Here's how the part is built. I have some questions about the finished solid (model axes, mm). Face numbers are marked on the shaded views. A direction names the side the tool comes from. Round coordinates to 2 decimals unless told otherwise and drop trailing zeros. Order: outer loops, then holes, each group sorted by start corner. A loop starts at its lowest first (then second) coordinate and runs counter-clockwise, first axis right, second up. Notation, with made-up numbers: (42.5, 76) -> (97.5, 76) arc R28 cw to (97.5, 108) -> close; hole circle Ø5 at (52.25, -14). An arc over 180 degrees is marked (long way). One line per item, written item: value.
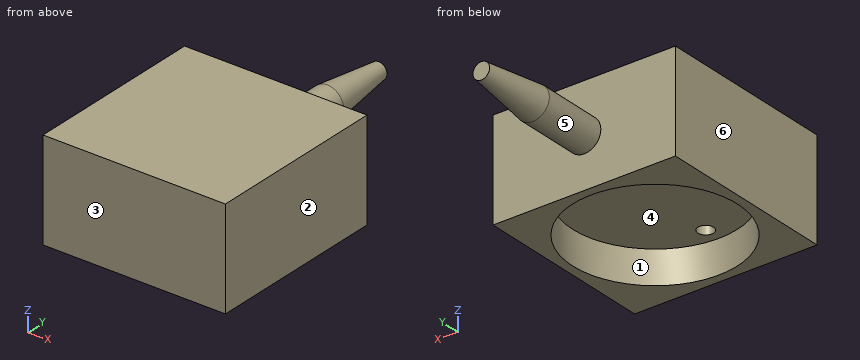
```python
from build123d import *

# Parameters (mm, degrees)
F2_W     = 69.85
F2_H     = 38.1
F3_DEPTH = 69.85
F4_R     = 3
F4_R_2   = 31.5
F5_DEPTH = 12.7
F6_DEPTH = 25.4


with BuildPart() as f1:
    # F0 (on Right) → F1 (revolve)
    with BuildSketch(Plane.YZ):
        Polygon((0, 6.35), (0, 0), (50.8, 0), (50.8, 3.175), (25.4, 6.35), align=None)
    revolve(axis=Axis((0, 25.4, 0), (0, 1, 0)))

    # F2 (on Front) → F3 (join)
    with BuildSketch(Plane.XZ):
        Rectangle(F2_W, F2_H)
    extrude(amount=F3_DEPTH)

    # F4 (on face) → F5 (cut)
    with BuildSketch(Plane(origin=(0, 0, -19.05), x_dir=(1, 0, 0), z_dir=(0, 0, -1))):
        with Locations((0, 59.925)):
            Circle(F4_R)
        with Locations((0, 34.925)):
            Circle(F4_R_2)
        with Locations((0, 59.925)):
            Circle(F4_R, mode=Mode.SUBTRACT)
    extrude(amount=-F5_DEPTH, mode=Mode.SUBTRACT)

    # F4 (on face) → F6 (cut)
    with BuildSketch(Plane(origin=(0, 0, -19.05), x_dir=(1, 0, 0), z_dir=(0, 0, -1))):
        with Locations((0, 59.925)):
            Circle(F4_R)
    extrude(amount=-F6_DEPTH, mode=Mode.SUBTRACT)


solid = f1.part
```
Q1. For P1, Ø4, axis at y = 13, z = 2.5, coming from the -X side; P2, Ø5, axis at y = 10.5, z = -1, coming from the +X side; P3, Ø5, axis at x = 17, z = 15, coming from the +Y side, each with a flat end and sliding along its axis, tell me the tip position at first contact or that it passes through.
Answers:
P1: x = -6.33
P2: x = 6.35
P3: y = 0
Q2. I want a section at C-C on y = -45. Write out the boundary of the cut face in (x, z) (3 decimals), then the cut area to 3 significant figures.
Answers:
outline: (-34.925, -19.05) -> (-29.845, -19.05) -> (-29.845, -6.35) -> (29.845, -6.35) -> (29.845, -19.05) -> (34.925, -19.05) -> (34.925, 19.05) -> (-34.925, 19.05) -> close
area: 1,900 mm2
Q3. I need wall thicknesses on line 1 along Y through (x, z) = (0, 0) (3 decimals); line 2 along X through (y, z) = (-35.5, -17) (3 decimals); line 3 along Y through (x, z) = (-6, 17). Which ranges of each line are inside material? Lowest first, please.
Answers:
line 1: -69.85 to -62.925, -56.925 to 50.8
line 2: -34.925 to -31.495, 31.495 to 34.925
line 3: -69.85 to 0
Q4. I want a section at A-A on x = 0. Write out the boundary of the cut face in (y, z) (3 decimals).
Answers:
outline: (-69.85, -19.05) -> (-66.425, -19.05) -> (-66.425, -6.35) -> (-62.925, -6.35) -> (-62.925, 6.35) -> (-56.925, 6.35) -> (-56.925, -6.35) -> (-3.425, -6.35) -> (-3.425, -19.05) -> (0, -19.05) -> (0, -6.35) -> (25.4, -6.35) -> (50.8, -3.175) -> (50.8, 3.175) -> (25.4, 6.35) -> (0, 6.35) -> (0, 19.05) -> (-69.85, 19.05) -> close
Q5. I want a section at D-D on x = -20. Write out the boundary of the cut face in (y, z).
Answers:
outline: (-69.85, -19.05) -> (-59.26, -19.05) -> (-59.26, -6.35) -> (-10.59, -6.35) -> (-10.59, -19.05) -> (0, -19.05) -> (0, 19.05) -> (-69.85, 19.05) -> close
Q6. If we mould it in two halves opening along X, with no side actions, what happens to the marked faces 1, 2 and 3? For each: pulls with the +X half, pulls with the -X half, needs draft (parallel to the pull), parting line crosses it, or undercut.
Answers:
face 1: undercut
face 2: pulls with the +X half
face 3: needs draft
Q7. Which directions (+Z, -Z, +X, -X, +Y, -Y) give clear straight access to the entire face, cutting with the end or side of a thin tool? Please do the marked faces 4, 5 and 6.
Answers:
face 4: -Z
face 5: +Y
face 6: +Z, -Z, -X, +Y, -Y
Q8. I want a section at B-B on z = -11.5. Write out the boundary of the cut face in (x, y) (3 decimals).
Answers:
outline: (-34.925, -69.85) -> (34.925, -69.85) -> (34.925, 0) -> (-34.925, 0) -> close; hole circle Ø63 at (0, -34.925)
